Input: part model. Units: mm. Frame: model coordinates. Face numbers are marked on the shaded views. A direction names the side the tool comes from. Round coordinates to 2 decimals unless told otherwise and drop trailing zeros. Write each loop counter-clockwise with the first axis right and the second up, starting at its lowest first coordinate (ties: lowest second). Pieces come first, ordered by that corner, then holes. Notation, with made-up numbers: (7, -12) - (64, -12) arc R24 ccw to (64, 11) - close; hole circle Ø1 at (82.5, 77.25). An arc over 180 degrees is marked (long way). One line per item, written item: value. Start each with the question number.
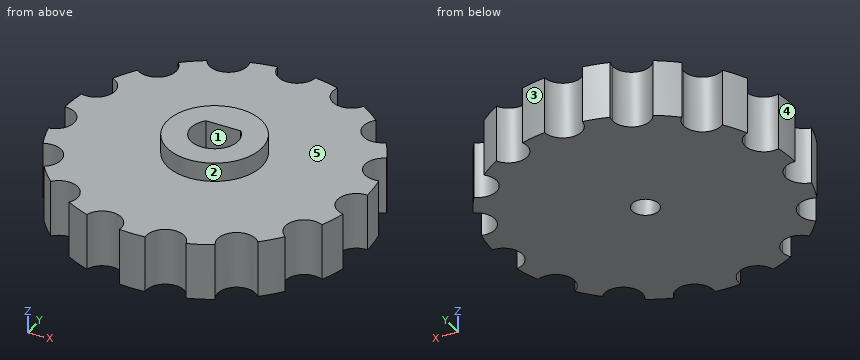
```python
from build123d import *

# Parameters (mm, degrees)
F0_R     = 12.5
F1_DEPTH = 15
F2_DEPTH = 20
F3_R     = 10
F3_R_2   = 3.5
F4_DEPTH = 5
F5_DEPTH = 15
F6_DEPTH = 20


with BuildPart() as f1:
    # F0 (on Top) → F1 (new body)
    with BuildSketch(Plane.XY):
        with BuildLine():
            ThreePointArc((38.948467, -9.111361), (34.808266, -3.658496), (39.991708, 0.814414))
            ThreePointArc((39.991708, 0.814414), (39.780876, 4.181139), (39.28712, 7.518126))
            ThreePointArc((39.28712, 7.518126), (33.286978, 10.815595), (36.202991, 17.010098))
            ThreePointArc((36.202991, 17.010098), (34.641016, 20), (32.832672, 22.847661))
            ThreePointArc((32.832672, 22.847661), (26.010069, 23.419571), (26.154448, 30.264581))
            ThreePointArc((26.154448, 30.264581), (23.51141, 32.36068), (20.701158, 34.226628))
            ThreePointArc((20.701158, 34.226628), (14.235783, 31.974091), (11.583563, 38.286043))
            ThreePointArc((11.583563, 38.286043), (8.316468, 39.125904), (4.990225, 39.6875))
            ThreePointArc((4.990225, 39.6875), (0, 35), (-4.990225, 39.6875))
            ThreePointArc((-4.990225, 39.6875), (-8.316468, 39.125904), (-11.583563, 38.286043))
            ThreePointArc((-11.583563, 38.286043), (-11.348617, 37.427958), (-11.269466, 36.541818))
            ThreePointArc((-11.269466, 36.541818), (-15.077505, 31.685973), (-20.701158, 34.226628))
            ThreePointArc((-20.701158, 34.226628), (-23.51141, 32.36068), (-26.154448, 30.264581))
            ThreePointArc((-26.154448, 30.264581), (-25.096715, 28.655102), (-24.725793, 26.765224))
            ThreePointArc((-24.725793, 26.765224), (-27.550293, 22.263314), (-32.832672, 22.847661))
            ThreePointArc((-32.832672, 22.847661), (-34.641016, 20), (-36.202991, 17.010098))
            ThreePointArc((-36.202991, 17.010098), (-33.907267, 15.171699), (-33.042261, 12.36068))
            ThreePointArc((-33.042261, 12.36068), (-34.9783, 8.409459), (-39.28712, 7.518126))
            ThreePointArc((-39.28712, 7.518126), (-39.780876, 4.181139), (-39.991708, 0.814414))
            ThreePointArc((-39.991708, 0.814414), (-36.320685, -0.571834), (-34.780876, -4.181139))
            ThreePointArc((-34.780876, -4.181139), (-35.962365, -7.408983), (-38.948467, -9.111361))
            ThreePointArc((-38.948467, -9.111361), (-38.042261, -12.36068), (-36.865496, -15.522089))
            ThreePointArc((-36.865496, -15.522089), (-32.006856, -15.750153), (-29.641016, -20))
            ThreePointArc((-29.641016, -20), (-30.234843, -22.363395), (-31.875271, -24.165411))
            ThreePointArc((-31.875271, -24.165411), (-29.725793, -26.765224), (-27.364904, -29.174681))
            ThreePointArc((-27.364904, -29.174681), (-21.818405, -27.656029), (-18.51141, -32.36068))
            ThreePointArc((-18.51141, -32.36068), (-18.710145, -33.756334), (-19.290551, -35.041043))
            ThreePointArc((-19.290551, -35.041043), (-16.269466, -36.541818), (-13.132672, -37.782707))
            ThreePointArc((-13.132672, -37.782707), (-7.638611, -34.172066), (-3.316468, -39.125904))
            ThreePointArc((-3.316468, -39.125904), (-3.329949, -39.492821), (-3.370319, -39.857759))
            ThreePointArc((-3.370319, -39.857759), (0, -40), (3.370319, -39.857759))
            ThreePointArc((3.370319, -39.857759), (7.276909, -34.235166), (13.132672, -37.782707))
            ThreePointArc((13.132672, -37.782707), (16.269466, -36.541818), (19.290551, -35.041043))
            ThreePointArc((19.290551, -35.041043), (20.572484, -28.315595), (27.364904, -29.174681))
            ThreePointArc((27.364904, -29.174681), (29.725793, -26.765224), (31.875271, -24.165411))
            ThreePointArc((31.875271, -24.165411), (30.310889, -17.5), (36.865496, -15.522089))
            ThreePointArc((36.865496, -15.522089), (38.042261, -12.36068), (38.948467, -9.111361))
        make_face()
        Circle(F0_R, mode=Mode.SUBTRACT)
    extrude(amount=F1_DEPTH)

    # F0 (on Top) → F2 (join)
    with BuildSketch(Plane.XY):
        Circle(F0_R)
        with BuildLine():
            ThreePointArc((4.582576, 4.25), (0, -6.25), (-4.582576, 4.25))
            Line((-4.582576, 4.25), (4.582576, 4.25))
        make_face(mode=Mode.SUBTRACT)
    extrude(amount=F2_DEPTH)

    # F3 (on Top) → F4 (join)
    with BuildSketch(Plane.XY):
        Circle(F3_R)
        Circle(F3_R_2, mode=Mode.SUBTRACT)
    extrude(amount=F4_DEPTH)



with BuildPart() as f5:
    # F0 (on Top) → F5 (new body)
    with BuildSketch(Plane.XY):
        with BuildLine():
            ThreePointArc((38.948467, -9.111361), (34.808266, -3.658496), (39.991708, 0.814414))
            ThreePointArc((39.991708, 0.814414), (39.780876, 4.181139), (39.28712, 7.518126))
            ThreePointArc((39.28712, 7.518126), (33.286978, 10.815595), (36.202991, 17.010098))
            ThreePointArc((36.202991, 17.010098), (34.641016, 20), (32.832672, 22.847661))
            ThreePointArc((32.832672, 22.847661), (26.010069, 23.419571), (26.154448, 30.264581))
            ThreePointArc((26.154448, 30.264581), (23.51141, 32.36068), (20.701158, 34.226628))
            ThreePointArc((20.701158, 34.226628), (14.235783, 31.974091), (11.583563, 38.286043))
            ThreePointArc((11.583563, 38.286043), (8.316468, 39.125904), (4.990225, 39.6875))
            ThreePointArc((4.990225, 39.6875), (0, 35), (-4.990225, 39.6875))
            ThreePointArc((-4.990225, 39.6875), (-8.316468, 39.125904), (-11.583563, 38.286043))
            ThreePointArc((-11.583563, 38.286043), (-11.348617, 37.427958), (-11.269466, 36.541818))
            ThreePointArc((-11.269466, 36.541818), (-15.077505, 31.685973), (-20.701158, 34.226628))
            ThreePointArc((-20.701158, 34.226628), (-23.51141, 32.36068), (-26.154448, 30.264581))
            ThreePointArc((-26.154448, 30.264581), (-25.096715, 28.655102), (-24.725793, 26.765224))
            ThreePointArc((-24.725793, 26.765224), (-27.550293, 22.263314), (-32.832672, 22.847661))
            ThreePointArc((-32.832672, 22.847661), (-34.641016, 20), (-36.202991, 17.010098))
            ThreePointArc((-36.202991, 17.010098), (-33.907267, 15.171699), (-33.042261, 12.36068))
            ThreePointArc((-33.042261, 12.36068), (-34.9783, 8.409459), (-39.28712, 7.518126))
            ThreePointArc((-39.28712, 7.518126), (-39.780876, 4.181139), (-39.991708, 0.814414))
            ThreePointArc((-39.991708, 0.814414), (-36.320685, -0.571834), (-34.780876, -4.181139))
            ThreePointArc((-34.780876, -4.181139), (-35.962365, -7.408983), (-38.948467, -9.111361))
            ThreePointArc((-38.948467, -9.111361), (-38.042261, -12.36068), (-36.865496, -15.522089))
            ThreePointArc((-36.865496, -15.522089), (-32.006856, -15.750153), (-29.641016, -20))
            ThreePointArc((-29.641016, -20), (-30.234843, -22.363395), (-31.875271, -24.165411))
            ThreePointArc((-31.875271, -24.165411), (-29.725793, -26.765224), (-27.364904, -29.174681))
            ThreePointArc((-27.364904, -29.174681), (-21.818405, -27.656029), (-18.51141, -32.36068))
            ThreePointArc((-18.51141, -32.36068), (-18.710145, -33.756334), (-19.290551, -35.041043))
            ThreePointArc((-19.290551, -35.041043), (-16.269466, -36.541818), (-13.132672, -37.782707))
            ThreePointArc((-13.132672, -37.782707), (-7.638611, -34.172066), (-3.316468, -39.125904))
            ThreePointArc((-3.316468, -39.125904), (-3.329949, -39.492821), (-3.370319, -39.857759))
            ThreePointArc((-3.370319, -39.857759), (0, -40), (3.370319, -39.857759))
            ThreePointArc((3.370319, -39.857759), (7.276909, -34.235166), (13.132672, -37.782707))
            ThreePointArc((13.132672, -37.782707), (16.269466, -36.541818), (19.290551, -35.041043))
            ThreePointArc((19.290551, -35.041043), (20.572484, -28.315595), (27.364904, -29.174681))
            ThreePointArc((27.364904, -29.174681), (29.725793, -26.765224), (31.875271, -24.165411))
            ThreePointArc((31.875271, -24.165411), (30.310889, -17.5), (36.865496, -15.522089))
            ThreePointArc((36.865496, -15.522089), (38.042261, -12.36068), (38.948467, -9.111361))
        make_face()
        Circle(F0_R, mode=Mode.SUBTRACT)
    extrude(amount=F5_DEPTH)


with BuildPart() as f1_1:
    add(f1.part)

    add(f5.part)  # F6 merges F5
    # F0 (on Top) → F6 (join)
    with BuildSketch(Plane.XY):
        Circle(F0_R)
        with BuildLine():
            ThreePointArc((4.582576, 4.25), (0, -6.25), (-4.582576, 4.25))
            Line((-4.582576, 4.25), (4.582576, 4.25))
        make_face(mode=Mode.SUBTRACT)
    extrude(amount=F6_DEPTH)


solid = f1_1.part
```
Q1. Cut plane A-A, the plane x = 0. Output: boundary loops of the cut face in (y, z).
Q2. Pull-direction query (Y, two-part tool) for the marked faces 1, 2 and 3; classes: pulls with the +Y half, pulls with the -Y half, needs draft (parallel to the pull), parting line crosses it, or undercut.
Q3. Material intervals for probe 1 along X at (y, z) = (33, 1); probe 2 along Y at (x, z) = (0, 16.5); probe 3 along Z at (x, y) = (8, -18), sorted ascending. Write a range as from..to.
Q4. Access query for the marked faces 4 and 5. Directions: +Z, -Z, +X, -X, +Y, -Y. A direction counts if a zero-diameter tool reaches every point of the face in a straight line with its end or side. Return the directions, or none.
Q5. Contact query for flat-ended pins moving along their axis: pin 1 Ø8 at (y, z) = (16, 6) entering from +X; pin 2 Ø3 at (x, z) = (-25, 8) entering from -Y; pin 3 Ø3 at (y, z) = (4.5, 12) entering from +X; pin 4 Ø5.5 at (x, y) = (0, 0) entering from -Z. Output: stop coordinate, or through.
Q6. Cut plane C-C, the plane z = 16.25. Output: boundary loops of the cut face in (x, y).
Q7. Cut plane B-B, the plane y = 2. Output: boundary loops of the cut face in (x, z).
Q8. Cut plane D-D, the plane x = -8. Output: boundary loops of the cut face in (y, z), and give its area (3 significant figures).
A:
1. outline: (-40, 0) - (-3.5, 0) - (-3.5, 5) - (-6.25, 5) - (-6.25, 20) - (-12.5, 20) - (-12.5, 15) - (-40, 15) - close; (3.5, 0) - (35, 0) - (35, 15) - (12.5, 15) - (12.5, 20) - (4.25, 20) - (4.25, 5) - (3.5, 5) - close
2. face 1: undercut
2. face 2: parting line crosses it
2. face 3: pulls with the +Y half
3. probe 1: x = -22.61..-19.8, -12.74..12.74, 19.8..22.61
3. probe 2: y = -12.5..-6.25, 4.25..12.5
3. probe 3: z = 0..15
4. face 4: +Z, -Z, -X, +Y
4. face 5: +Z
5. pin 1: stops at x = 36.2
5. pin 2: stops at y = -28.35
5. pin 3: stops at x = 39.89
5. pin 4: passes through
6. outline: circle Ø25 at (0, 0); hole (-4.58, 4.25) arc R6.25 ccw (long way) to (4.58, 4.25) - close
7. outline: (-39.95, 0) - (-2.87, 0) - (-2.87, 5) - (-5.92, 5) - (-5.92, 20) - (-12.34, 20) - (-12.34, 15) - (-39.95, 15) - close; (2.87, 0) - (39.95, 0) - (39.95, 15) - (12.34, 15) - (12.34, 20) - (5.92, 20) - (5.92, 5) - (2.87, 5) - close
8. outline: (-34.14, 0) - (39.19, 0) - (39.19, 15) - (9.6, 15) - (9.6, 20) - (-9.6, 20) - (-9.6, 15) - (-34.14, 15) - close
8. area: 1,200 mm²
